Verification items for the finished model (mm, model axes). Face numbers are marked on the shaded views. Coordinates: 2 decimals unless noted, no trailing zeros. Order: outer loops, then holes, each group sorted by start corner. A loop starts at its lowest first (then second) coordinate and runs counter-clockwise, first axis right, second up. Notation, with made-up numbers: (-5, 8) -> (48, 8) arc R17 cw to (48, 39) -> close; hole circle Ø6 at (13.5, 37.5). An arc over 180 degrees is marked (long way). Write item = value, one per line. Start each with the question number.
1. Cross-section at A-A on y = 0. Record the cut outline in (x, z).
2. Cross-section at C-C on y = -20. Record the cut outline in (x, z).
3. Cross-section at D-D on z = 6. Record the cut outline in (x, y), plus the area to 3 significant figures.
4. Thickness scan on line 1 along Y through (x, z) = (0, 15.5); line 2 along Y through (x, z) = (0, 6.5); line 3 along Z through (x, y) = (5, -37.5). Record the ranges inside material, lowest first. Write a range as from..to.
5. Release check for a two-part mould opening along X. For the marked faces 1, 2, 3 and 4 record: +X half, -X half, draft (parallel to the pull), parting line (faces both ways), or undercut.
6. Cross-section at B-B on x = -10. Record the cut outline in (y, z), plus the area to 3 significant figures.
7. Go/stop test with flat-tipped pins: P1, Ø3, axis at y = -6, z = 7.5, coming from the +X side; P2, Ø2, axis at x = 18.5, y = 1.5, coming from the -Z side; P3, Ø1.5, axis at x = -2.5, z = 14, coming from the +Y side. Record where each tip stops, or that it passes through.
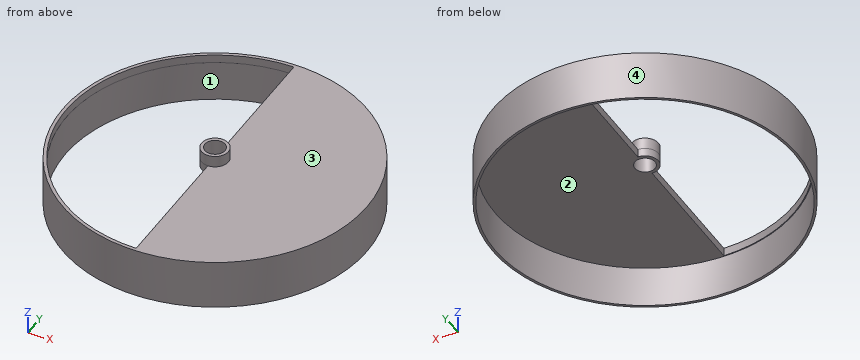
from build123d import *

# Parameters (mm, degrees)
F0_R          = 46.5
F1_DEPTH      = 15.24
F2_R          = 45.75
F3_DEPTH      = 12.7
F4_R          = 4.1
F5_DEPTH      = 3.53
F5_DEPTH_BACK = 1
F7_R          = 3.1
F8_DEPTH      = 18.771
F9_DEPTH      = 15.241


# Not quite as in the source:
# - after a boolean that leaves OpenCascade's solid faulty, fix() repairs it


with BuildPart() as f1:
    # F0 (on Top) → F1 (new body)
    with BuildSketch(Plane.XY):
        Circle(F0_R)
    extrude(amount=F1_DEPTH)

    # F2 (on Top) → F3 (cut)
    with BuildSketch(Plane.XY):
        Circle(F2_R)
    extrude(amount=F3_DEPTH, mode=Mode.SUBTRACT)

    # F4 (on face) → F5 (join, two sides)
    with BuildSketch(Plane.XY.offset(15.24)) as f5_sk:
        Circle(F4_R)
    extrude(amount=F5_DEPTH)
    extrude(f5_sk.sketch, amount=-F5_DEPTH_BACK)

    # F7 (on face) → F8 (cut, through all)
    with BuildSketch(Plane.XY.offset(18.77)):
        Circle(F7_R)
    extrude(amount=-F8_DEPTH, mode=Mode.SUBTRACT)

    # F6 (on face) → F9 (cut, through all)
    with BuildSketch(Plane.XY.offset(15.24)):
        with BuildLine():
            Line((0, 4.1), (0, 45.5))
            ThreePointArc((0, 45.5), (-45.5, 0), (0, -45.5))
            Line((0, -45.5), (0, -4.1))
            ThreePointArc((0, -4.1), (-4.1, 0), (0, 4.1))
        make_face()
    extrude(amount=-F9_DEPTH, mode=Mode.SUBTRACT)

    add(f1.part.fix(), mode=Mode.REPLACE)


solid = f1.part
Worked out:
q1.outline = (-46.5, 0) -> (-45.75, 0) -> (-45.75, 12.7) -> (-45.5, 12.7) -> (-45.5, 15.24) -> (-46.5, 15.24) -> close; (-4.1, 12.7) -> (-3.1, 12.7) -> (-3.1, 18.77) -> (-4.1, 18.77) -> close; (3.1, 12.7) -> (45.75, 12.7) -> (45.75, 0) -> (46.5, 0) -> (46.5, 15.24) -> (4.1, 15.24) -> (4.1, 18.77) -> (3.1, 18.77) -> close
q2.outline = (-41.98, 0) -> (-41.15, 0) -> (-41.15, 12.7) -> (-40.87, 12.7) -> (-40.87, 15.24) -> (-41.98, 15.24) -> close; (0, 12.7) -> (41.15, 12.7) -> (41.15, 0) -> (41.98, 0) -> (41.98, 15.24) -> (0, 15.24) -> close
q3.outline = circle Ø93 at (0, 0); hole circle Ø91.5 at (0, 0)
q3.area = 217 mm²
q4.line_1 = -4.1..-3.1, 3.1..4.1
q4.line_2 = -46.5..-45.75, 45.75..46.5
q4.line_3 = 12.7..15.24
q5.face_1 = undercut
q5.face_2 = undercut
q5.face_3 = draft
q5.face_4 = parting line
q6.outline = (-45.41, 0) -> (-44.64, 0) -> (-44.64, 12.7) -> (-44.39, 12.7) -> (-44.39, 15.24) -> (-45.41, 15.24) -> close; (44.39, 12.7) -> (44.64, 12.7) -> (44.64, 0) -> (45.41, 0) -> (45.41, 15.24) -> (44.39, 15.24) -> close
q6.area = 24.7 mm²
q7.P1 = 46.28
q7.P2 = 12.7
q7.P3 = 46.47
